from build123d import *

# Parameters (mm, degrees)
SKETCH1_W                    = 110
SKETCH1_H                    = 200
SKETCH1_W_2                  = 70
SKETCH1_H_2                  = 120
BASE_FLANGE1_DEPTH           = 0.7366
EDGE_FLANGE1_STRIP_W         = 4.4196
EDGE_FLANGE1_STRIP_H         = 0.7366
EDGE_FLANGE1_STRIP_CUT_DEPTH = 200
EDGE_FLANGE1_DEPTH           = 200
EDGE_FLANGE2_STRIP_W         = 4.4196
EDGE_FLANGE2_STRIP_H         = 0.7366
EDGE_FLANGE2_STRIP_CUT_DEPTH = 200
EDGE_FLANGE2_DEPTH           = 200
EDGE_FLANGE3_STRIP_W         = 4.4196
EDGE_FLANGE3_STRIP_H         = 0.7366
EDGE_FLANGE3_STRIP_CUT_DEPTH = 108.5268
EDGE_FLANGE3_DEPTH           = 108.5268
EDGE_FLANGE3_START           = 0.7366
EDGE_FLANGE3_FLAT_DEPTH      = 0.7366
EDGE_FLANGE4_STRIP_W         = 4.4196
EDGE_FLANGE4_STRIP_H         = 0.7366
EDGE_FLANGE4_STRIP_CUT_DEPTH = 108.5268
EDGE_FLANGE4_DEPTH           = 108.5268
EDGE_FLANGE4_START           = 0.7366
EDGE_FLANGE4_FLAT_DEPTH      = 0.7366
CUT_EXTRUDE2_DEPTH           = 289.797370967
CUT_EXTRUDE3_START           = -0.7366
CUT_EXTRUDE3_DEPTH           = 0.7366
CUT_EXTRUDE6_DEPTH           = 800.082459726
CUT_EXTRUDE6_DEPTH_BACK      = 800.082459726
SKETCH53_R                   = 2.2
SKETCH53_R_2                 = 2.199999998


# Read off the part's stored shape, not the designer's step: Cut-Extrude3
# Sheet-metal steps are written as plain solids
with BuildPart() as part:
    # Sketch1 → Base-Flange1 (new body)
    with BuildSketch(Plane(origin=(0, 0, 0), x_dir=(1, 0, 0), z_dir=(0, 1, 0))):
        Rectangle(SKETCH1_W, SKETCH1_H)
        Rectangle(SKETCH1_W_2, SKETCH1_H_2, mode=Mode.SUBTRACT)
    extrude(amount=-BASE_FLANGE1_DEPTH)

    # Edge-Flange1 strip (across the edge) → Edge-Flange1 strip cut (cut)
    with BuildSketch(Plane(origin=(-55, 0, -100), x_dir=(1, 0, 0), z_dir=(0, 0, 1))):
        with Locations((-1.4732, -0.3683)):
            Rectangle(EDGE_FLANGE1_STRIP_W, EDGE_FLANGE1_STRIP_H)
    extrude(amount=EDGE_FLANGE1_STRIP_CUT_DEPTH, mode=Mode.SUBTRACT)

    # Edge-Flange1 section (across the edge) → Edge-Flange1 (add)
    with BuildSketch(Plane(origin=(-55, 0, -100), x_dir=(1, 0, 0), z_dir=(0, 0, 1))):
        with BuildLine():
            Line((-0.7366, 0.7366), (-0.7366, 199.2634))
            Line((-0.7366, 199.2634), (0, 199.2634))
            Line((0, 199.2634), (0, 0.7366))
            ThreePointArc((0, 0.7366), (0.215745145, 0.215745145), (0.7366, 0))
            Line((0.7366, 0), (0.7366, -0.7366))
            ThreePointArc((0.7366, -0.7366), (-0.30510971, -0.30510971), (-0.7366, 0.7366))
        make_face()
    extrude(amount=EDGE_FLANGE1_DEPTH)

    # Edge-Flange2 strip (across the edge) → Edge-Flange2 strip cut (cut)
    with BuildSketch(Plane(origin=(55, 0, 100), x_dir=(-1, 0, 0), z_dir=(0, 0, -1))):
        with Locations((-1.4732, -0.3683)):
            Rectangle(EDGE_FLANGE2_STRIP_W, EDGE_FLANGE2_STRIP_H)
    extrude(amount=EDGE_FLANGE2_STRIP_CUT_DEPTH, mode=Mode.SUBTRACT)

    # Edge-Flange2 section (across the edge) → Edge-Flange2 (add)
    with BuildSketch(Plane(origin=(55, 0, 100), x_dir=(-1, 0, 0), z_dir=(0, 0, -1))):
        with BuildLine():
            Line((-0.7366, 0.7366), (-0.7366, 99.2634))
            Line((-0.7366, 99.2634), (0, 99.2634))
            Line((0, 99.2634), (0, 0.7366))
            ThreePointArc((0, 0.7366), (0.215745145, 0.215745145), (0.7366, 0))
            Line((0.7366, 0), (0.7366, -0.7366))
            ThreePointArc((0.7366, -0.7366), (-0.30510971, -0.30510971), (-0.7366, 0.7366))
        make_face()
    extrude(amount=EDGE_FLANGE2_DEPTH)

    # Edge-Flange3 strip (across the edge) → Edge-Flange3 strip cut (cut)
    with BuildSketch(Plane(origin=(54.2634, 0, -100), x_dir=(0, 0, 1), z_dir=(-1, 0, 0))):
        with Locations((-1.4732, -0.3683)):
            Rectangle(EDGE_FLANGE3_STRIP_W, EDGE_FLANGE3_STRIP_H)
    extrude(amount=EDGE_FLANGE3_STRIP_CUT_DEPTH, mode=Mode.SUBTRACT)

    # Edge-Flange3 bend section (across the edge) → Edge-Flange3 (add)
    with BuildSketch(Plane(origin=(54.2634, 0, -100), x_dir=(0, 0, 1), z_dir=(-1, 0, 0))):
        with BuildLine():
            Line((-0.7366, 0.7366), (0, 0.7366))
            ThreePointArc((0, 0.7366), (0.215745145, 0.215745145), (0.7366, 0))
            Line((0.7366, 0), (0.7366, -0.7366))
            ThreePointArc((0.7366, -0.7366), (-0.30510971, -0.30510971), (-0.7366, 0.7366))
        make_face()
    extrude(amount=EDGE_FLANGE3_DEPTH)

    # Edge-Flange3 profile (on flange) → Edge-Flange3 flat (add)
    with BuildSketch(Plane(origin=(0, 0, -100), x_dir=(-1, 0, 0), z_dir=(0, 0, -1)).offset(EDGE_FLANGE3_START)):
        Polygon((-54.2634, 115), (-54.2634, 0.7366), (54.2634, 0.7366), (54.2634, 199.2634), align=None)
    extrude(amount=-EDGE_FLANGE3_FLAT_DEPTH)

    # Edge-Flange4 strip (across the edge) → Edge-Flange4 strip cut (cut)
    with BuildSketch(Plane(origin=(-54.2634, 0, 100), x_dir=(0, 0, -1), z_dir=(1, 0, 0))):
        with Locations((-1.4732, -0.3683)):
            Rectangle(EDGE_FLANGE4_STRIP_W, EDGE_FLANGE4_STRIP_H)
    extrude(amount=EDGE_FLANGE4_STRIP_CUT_DEPTH, mode=Mode.SUBTRACT)

    # Edge-Flange4 bend section (across the edge) → Edge-Flange4 (add)
    with BuildSketch(Plane(origin=(-54.2634, 0, 100), x_dir=(0, 0, -1), z_dir=(1, 0, 0))):
        with BuildLine():
            Line((-0.7366, 0.7366), (0, 0.7366))
            ThreePointArc((0, 0.7366), (0.215745145, 0.215745145), (0.7366, 0))
            Line((0.7366, 0), (0.7366, -0.7366))
            ThreePointArc((0.7366, -0.7366), (-0.30510971, -0.30510971), (-0.7366, 0.7366))
        make_face()
    extrude(amount=EDGE_FLANGE4_DEPTH)

    # Edge-Flange4 profile (on flange) → Edge-Flange4 flat (add)
    with BuildSketch(Plane.XY.offset(100).offset(EDGE_FLANGE4_START)):
        Polygon((-54.2634, 199.2634), (-54.2634, 0.7366), (54.2634, 0.7366), (54.2634, 115), align=None)
    extrude(amount=-EDGE_FLANGE4_FLAT_DEPTH)

    # Sketch24 → Cut-Extrude2 (cut, through all)
    with BuildSketch(Plane(origin=(0, 0, -100.7366), x_dir=(-1, 0, 0), z_dir=(0, 0, -1))):
        Polygon((-28.519875042, 107.808063094), (31.460124178, 107.808063094), (31.460124178, 158.533542729), align=None)
        Polygon((-28.150641863, 10.732953924), (31.829357358, 10.732953924), (31.829357358, 61.45843356), align=None)
        Polygon((31.713150602, 88.173102361), (-28.636081798, 88.173102361), (-28.636081798, 37.135359798), align=None)
    extrude(amount=-CUT_EXTRUDE2_DEPTH, mode=Mode.SUBTRACT)

    # Cut-Extrude3 outline → Cut-Extrude3 (cut)
    with BuildSketch(Plane(origin=(55.7366, 0, 0), x_dir=(0, 0, -1), z_dir=(1, 0, 0)).offset(CUT_EXTRUDE3_START)):
        with BuildLine():
            Line((-87.713422796, 42.053472661), (-6.797155753, 39.040000774))
            add(Edge.make_bspline(
                [(-6.797155753, 39.040000774), (-87.713422796, 42.053472661), (67.110125935, 80.068334048), (60.312641059, 39.424036929), (22.052524279, 39.424036929)],
                knots=[0, 0, 0, 0, 0, 1, 1, 1, 1, 1], degree=4))
            Line((22.052524279, 39.424036929), (60.312641059, 39.424036929))
            ThreePointArc((60.312641059, 39.424036929), (80.917037974, 56.86865569), (67.110125935, 80.068334048))
            Line((67.110125935, 80.068334048), (-87.713422796, 42.053472661))
        make_face()
    extrude(amount=CUT_EXTRUDE3_DEPTH, mode=Mode.SUBTRACT)

    # Sketch53 → Cut-Extrude6 (cut, two sides: drawn at the far end of the back side and taken through both)
    with BuildSketch(Plane(origin=(344.115063699, 0, 561.793038506), x_dir=(-1, 0, 0), z_dir=(0, 1, 0)).offset(-CUT_EXTRUDE6_DEPTH_BACK)):
        with Locations(Location((392.463649434, -480.956438506, 0), (0, 0, 90))):
            Circle(SKETCH53_R)
        with Locations(Location((392.463649434, -465.956438506, 0), (0, 0, 90))):
            Circle(SKETCH53_R)
        with Locations(Location((362.463649434, -473.456438506, 0), (0, 0, 90))):
            Circle(SKETCH53_R)
        with Locations(Location((292.463649434, -480.956438506, 0), (0, 0, 90))):
            Circle(SKETCH53_R)
        with Locations(Location((292.463649434, -465.956438506, 0), (0, 0, 90))):
            Circle(SKETCH53_R)
        with Locations(Location((322.463649434, -473.456438506, 0), (0, 0, 90))):
            Circle(SKETCH53_R)
        with Locations(Location((294.03158687, -636.983238506, 0), (0, 0, 90))):
            Circle(SKETCH53_R_2)
        with Locations(Location((324.69158687, -646.983238506, 0), (0, 0, 90))):
            Circle(SKETCH53_R_2)
        with Locations(Location((346.36158687, -636.983238506, 0), (0, 0, 90))):
            Circle(SKETCH53_R_2)
        with Locations(Location((368.028253537, -646.983238506, 0), (0, 0, 90))):
            Circle(SKETCH53_R_2)
        with Locations(Location((389.694920203, -636.983238506, 0), (0, 0, 90))):
            Circle(SKETCH53_R_2)
    extrude(amount=CUT_EXTRUDE6_DEPTH + CUT_EXTRUDE6_DEPTH_BACK, mode=Mode.SUBTRACT)


solid = part.part
Read the model definition and answer for the solid it produces. Units are mm, in the model's axes. A direction names the side the tool comes from. Coordinates: 2 decimals unless noted, no trailing zeros. Loops run counter-clockwise (first coordinate to the right, second up) from the corner with the lowest first, then second, coordinate; pieces in that order, holes last.
Q1. The part is cut by section D-D on y = 71.5. Write down the section's boundary in (x, z).
Q2. Each of these flat-tipped pins is pushed along its axis until it touches: pin 1 Ø5 at (x, z) = (-48.35, 95.84) entering from +Y; pin 2 Ø3.5 at (x, z) = (-2.25, -75.19) entering from +Y. Where does it stop, or does it pass through?
Q3. The part is cut by section B-B on y = 145. Write down the section's boundary in (x, z), and give its area (3 significant figures).
Q4. The part is cut by section A-A on x = 32.5. Write down the section's boundary in (y, z).
Q5. The mould has two halves that part along Z. Classify faces 1 (the face through (-13, 101, 100)), 2 (the face through (-1.12, 62.3, -100.37)), 3 (the face through (-13, 101, 100.737)): +Z half, -Z half, draft (parallel to the pull), parting line (faces both ways), or undercut.
Q6. Which of the six approach directions +Z, -Z, +X, -X, +Y, -Y give full straight-line access (tool end or side, diameter ignored) to faces 4 (the face through (55.363, 61.327, 9.218)), 5 (the face through (-55, 101, -1)), 6 (the face through (-1.89, 133.526, -100.373)), 7 (the face through (-37, 0, -1))?
Q7. The part is cut by section C-C on z = 44.5. Write down the section's boundary in (x, y).
Q8. Consider probe 1 along Z at (x, y) = (-14.5, 59); probe 2 along X at (y, z) = (57.5, 88); probe 3 along Y at (x, z) = (-11, 66). Determine where each line is inside the solid, lowest interval first.
Results below:
1. outline: (-55.74, -100) - (-55, -100) - (-55, 100) - (-55.74, 100) - close; (-54.26, -100.74) - (-12, -100.74) - (-12, -100) - (-54.26, -100) - close; (-54.26, 100) - (-12, 100) - (-12, 100.74) - (-54.26, 100.74) - close; (28.64, -100.74) - (54.26, -100.74) - (54.26, -100) - (28.64, -100) - close; (28.64, 100) - (54.26, 100) - (54.26, 100.74) - (28.64, 100.74) - close; (55, -100) - (55.74, -100) - (55.74, -77.96) - (55, -77.96) - close; (55, -32.21) - (55.74, -32.21) - (55.74, 100) - (55, 100) - close
2. pin 1: stops at y = 0
2. pin 2: passes through
3. outline: (-55.74, -100) - (-55, -100) - (-55, 100) - (-55.74, 100) - close; (-54.26, -100.74) - (-31.46, -100.74) - (-31.46, -100) - (-54.26, -100) - close; (-54.26, 100) - (-31.46, 100) - (-31.46, 100.74) - (-54.26, 100.74) - close; (-15.46, -100.74) - (15.62, -100.74) - (15.62, -100) - (-15.46, -100) - close; (-15.46, 100) - (15.62, 100) - (15.62, 100.74) - (-15.46, 100.74) - close
3. area: 227 mm2
4. outline: (-0.74, -99.26) arc R1.47 ccw to (0.74, -100.74) - (131.9, -100.74) - (131.9, -100) - (0.74, -100) arc R0.74 cw to (0, -99.26) - (0, -60) - (-0.74, -60) - close; (-0.74, 60) - (0, 60) - (0, 99.26) arc R0.74 cw to (0.74, 100) - (131.9, 100) - (131.9, 100.74) - (0.74, 100.74) arc R1.47 ccw to (-0.74, 99.26) - close
5. face 1: undercut
5. face 2: draft
5. face 3: +Z half
6. face 4: +X
6. face 5: +Z, -Z, +Y
6. face 6: +Z, -Z
6. face 7: +Y
7. outline: (-55.74, 0.74) arc R1.47 ccw to (-54.26, -0.74) - (-35, -0.74) - (-35, 0) - (-54.26, 0) arc R0.74 cw to (-55, 0.74) - (-55, 199.26) - (-55.74, 199.26) - close; (35, -0.74) - (54.26, -0.74) arc R1.47 ccw to (55.74, 0.74) - (55.74, 40.44) - (55, 40.44) - (55, 0.74) arc R0.74 cw to (54.26, 0) - (35, 0) - close; (55, 52.66) - (55.74, 52.66) - (55.74, 99.26) - (55, 99.26) - close
8. probe 1: z = -100.74 to -100, 100 to 100.74
8. probe 2: x = -55.74 to -55, 55 to 55.74
8. probe 3: y = -0.74 to 0
